from build123d import *

# Parameters (mm, degrees)
FLANGE_BASE1_DEPTH             = 3
CORTE_EXTRUS_O1_DEPTH          = 3
ARESTA_FLANGE4_STRIP_W         = 13.4732
ARESTA_FLANGE4_STRIP_H         = 3
ARESTA_FLANGE4_STRIP_CUT_DEPTH = 18.4
ARESTA_FLANGE4_DEPTH           = 18.4
ESBO_O47_W                     = 14.5
ESBO_O47_H                     = 15
RESSALTO_EXTRUS_O1_DEPTH       = 3
FILETE1_R                      = 5
ESBO_O48_W                     = 14.5
ESBO_O48_H                     = 15
RESSALTO_EXTRUS_O2_DEPTH       = 3
FILETE2_R                      = 5
FILETE3_R                      = 2
CORTE_EXTRUS_O5_DEPTH          = 42.850190918
CORTE_EXTRUS_O6_DEPTH          = 3


# Sheet-metal steps are written as plain solids
with BuildPart() as part:
    # Esboço1 → Flange-base1 (new body)
    with BuildSketch(Plane.XY):
        Polygon((-14.370772566, 2.693459119), (-4.370772566, 2.693459119), (-4.370772566, 5.943459119), (14.029227434, 5.943459119), (14.029227434, 2.693459119), (21.029227434, 2.693459119), (21.029227434, -4.306540881), (-14.370772566, -4.306540881), align=None)
    extrude(amount=-FLANGE_BASE1_DEPTH)

    # Esboço8 → Corte-extrusão1 (cut)
    with BuildSketch(Plane.XY):
        with BuildLine():
            Line((-10.260200759, 1.193459119), (-2.260200759, 1.193459119))
            ThreePointArc((-2.260200759, 1.193459119), (-0.260200759, -0.806540881), (-2.260200759, -2.806540881))
            Line((-2.260200759, -2.806540881), (-10.260200759, -2.806540881))
            ThreePointArc((-10.260200759, -2.806540881), (-12.260200759, -0.806540881), (-10.260200759, 1.193459119))
        make_face()
        with BuildLine():
            Line((8.88097681, 1.193459119), (17.620096532, 1.193459119))
            ThreePointArc((17.620096532, 1.193459119), (19.620096532, -0.806540881), (17.620096532, -2.806540881))
            Line((17.620096532, -2.806540881), (8.88097681, -2.806540881))
            ThreePointArc((8.88097681, -2.806540881), (6.88097681, -0.806540881), (8.88097681, 1.193459119))
        make_face()
    extrude(amount=-CORTE_EXTRUS_O1_DEPTH, mode=Mode.SUBTRACT)

    # Aresta-Flange4 strip (across the edge) → Aresta-Flange4 strip cut (cut)
    with BuildSketch(Plane(origin=(14.029227434, 5.943459119, 0), x_dir=(0, -1, 0), z_dir=(-1, 0, 0))):
        with Locations((-6, -1.5)):
            Rectangle(ARESTA_FLANGE4_STRIP_W, ARESTA_FLANGE4_STRIP_H)
    extrude(amount=ARESTA_FLANGE4_STRIP_CUT_DEPTH, mode=Mode.SUBTRACT)

    # Aresta-Flange4 section (across the edge) → Aresta-Flange4 (add)
    with BuildSketch(Plane(origin=(14.029227434, 5.943459119, 0), x_dir=(0, -1, 0), z_dir=(-1, 0, 0))):
        with BuildLine():
            Line((-3, 0.7366), (-3, 22.5))
            Line((-3, 22.5), (0, 22.5))
            Line((0, 22.5), (0, 0.7366))
            ThreePointArc((0, 0.7366), (0.215745145, 0.215745145), (0.7366, 0))
            Line((0.7366, 0), (0.7366, -3))
            ThreePointArc((0.7366, -3), (-1.905575199, -1.905575199), (-3, 0.7366))
        make_face()
    extrude(amount=ARESTA_FLANGE4_DEPTH)

    # Esboço47 → Ressalto-extrusão1 (add)
    with BuildSketch(Plane(origin=(14.029227434, 0, 0), x_dir=(0, 0, -1), z_dir=(1, 0, 0))):
        with Locations((-15.25, 13.443459119)):
            Rectangle(ESBO_O47_W, ESBO_O47_H)
    extrude(amount=-RESSALTO_EXTRUS_O1_DEPTH)

    # Filete1
    filete1_edges = [part.edges().sort_by_distance(p)[0] for p in [
        (12.529227434, 20.943459119, 22.5),
        (12.529227434, 8.943459119, 8),
        (12.529227434, 20.943459119, 8),
    ]]
    fillet(filete1_edges, radius=FILETE1_R)

    # Esboço48 → Ressalto-extrusão2 (add)
    with BuildSketch(Plane.ZY.offset(4.370772566)):
        with Locations((15.25, 13.443459119)):
            Rectangle(ESBO_O48_W, ESBO_O48_H)
    extrude(amount=-RESSALTO_EXTRUS_O2_DEPTH)

    # Filete2
    filete2_edges = [part.edges().sort_by_distance(p)[0] for p in [
        (-2.870772566, 20.943459119, 22.5),
        (-2.870772566, 8.943459119, 8),
        (-2.870772566, 20.943459119, 8),
    ]]
    fillet(filete2_edges, radius=FILETE2_R)

    # Filete3
    filete3_edges = [part.edges().sort_by_distance(p)[0] for p in [
        (21.029227434, -4.306540881, -1.5),
        (-14.370772566, -4.306540881, -1.5),
        (-14.370772566, 2.693459119, -1.5),
        (-4.370772566, 2.693459119, -1.5),
        (14.029227434, 2.693459119, -1.5),
        (21.029227434, 2.693459119, -1.5),
    ]]
    fillet(filete3_edges, radius=FILETE3_R)

    # Esboço49 → Corte-extrusão5 (cut, through all)
    with BuildSketch(Plane(origin=(14.029227434, 0, 0), x_dir=(0, 0, -1), z_dir=(1, 0, 0))):
        with BuildLine():
            Line((-18.2, 11.175198381), (-12.3, 11.175198381))
            ThreePointArc((-12.3, 11.175198381), (-10.885786438, 11.760984819), (-10.3, 13.175198381))
            Line((-10.3, 13.175198381), (-10.3, 17.289297618))
            ThreePointArc((-10.3, 17.289297618), (-10.885786438, 18.70351118), (-12.3, 19.289297618))
            Line((-12.3, 19.289297618), (-18.2, 19.289297618))
            ThreePointArc((-18.2, 19.289297618), (-19.614213562, 18.70351118), (-20.2, 17.289297618))
            Line((-20.2, 17.289297618), (-20.2, 13.175198381))
            ThreePointArc((-20.2, 13.175198381), (-19.614213562, 11.760984819), (-18.2, 11.175198381))
        make_face()
    extrude(amount=-CORTE_EXTRUS_O5_DEPTH, mode=Mode.SUBTRACT)

    # Esboço50 → Corte-extrusão6 (cut)
    with BuildSketch(Plane.XZ.offset(-5.943459119)):
        with BuildLine():
            Line((1.629227434, 19.2366), (8.029227434, 19.2366))
            ThreePointArc((8.029227434, 19.2366), (9.443440996, 18.650813562), (10.029227434, 17.2366))
            Line((10.029227434, 17.2366), (10.029227434, 5.2366))
            ThreePointArc((10.029227434, 5.2366), (9.443440996, 3.822386438), (8.029227434, 3.2366))
            Line((8.029227434, 3.2366), (1.629227434, 3.2366))
            ThreePointArc((1.629227434, 3.2366), (0.215013871, 3.822386438), (-0.370772566, 5.2366))
            Line((-0.370772566, 5.2366), (-0.370772566, 17.2366))
            ThreePointArc((-0.370772566, 17.2366), (0.215013871, 18.650813562), (1.629227434, 19.2366))
        make_face()
    extrude(amount=-CORTE_EXTRUS_O6_DEPTH, mode=Mode.SUBTRACT)


solid = part.part
Design review of the part built by this model. Coordinates are the model's own, in mm. A direction names the side the tool comes from. Coordinates: 2 decimals unless noted, no trailing zeros. Loops run counter-clockwise (first coordinate to the right, second up) from the corner with the lowest first, then second, coordinate; pieces in that order, holes last. Notation, with made-up numbers: M 50.5,20.25 L 91.5,20.25 A23 ccw 91.5,38.25 Z; hole C 64.5,42.25 d5. An arc over 180 degrees is marked long. Use one line per item in the form item = value.
(1) Consider section B-B (z = 15). Write out the cut boundary in (x, y).
Return value:
outline = M -4.37,5.94 L -0.37,5.94 L -0.37,8.94 L -1.37,8.94 L -1.37,11.18 L -4.37,11.18 Z; M -4.37,19.29 L -1.37,19.29 L -1.37,20.94 L -4.37,20.94 Z; M 10.03,5.94 L 14.03,5.94 L 14.03,11.18 L 11.03,11.18 L 11.03,8.94 L 10.03,8.94 Z; M 11.03,19.29 L 14.03,19.29 L 14.03,20.94 L 11.03,20.94 Z
(2) Consider section C-C (x = 4). Write out the cut boundary in (y, z).
Return value:
outline = M -4.31,-3 L 5.21,-3 A3.74 ccw 8.94,0.74 L 8.94,3.24 L 5.94,3.24 L 5.94,0.74 A0.74 cw 5.21,0 L -4.31,0 Z; M 5.94,19.24 L 8.94,19.24 L 8.94,22.5 L 5.94,22.5 Z
(3) Draft analysis for pull direction Z (two halves, no side actions). For faces 6 (the face through (21.029, -1, -1)), 7 (the face through (10.029, 7, 11)), 8 (the face through (12.508, 10.447, 6.574)), state which applies: pulls with the +Z half, pulls with the -Z half, needs draft (parallel to the pull), parting line crosses it, or undercut.
Return value:
face_6 = needs draft
face_7 = undercut
face_8 = pulls with the -Z half
(4) Clearance check with flat-ended pins moving along their axes: P1, Ø5, axis at y = 6.5, z = 2, coming from the +X side; P2, Ø10, axis at x = 8, z = 8.5, coming from the +Y side; P3, Ø10, axis at x = 11, z = 13.5, coming from the -Y side; P4, Ø14.5, axis at x = 3.5, z = 7, coming from the -Y side. State where each tip first meets the part, or that it passes through.
Return value:
P1 = 14.03
P2 = 20.92
P3 = 5.94
P4 = -4.31
(5) For faces 1 (the face through (-6, -2.807, -1)), 2 (the face through (11.029, 11, 15)), 3 (the face through (13, 15, 10.3)), 4 (the face through (9.46, 7.42, 3.84)), 5 (the face through (-9, 2.693, -1)), list the 3-axis set-ups (+Z, -Z, +X, -X, +Y, -Y) from which the entire face can be reached by the end or side of a thin tool; tool diameter is ignored.
Return value:
face_1 = +Z, -Z
face_2 = +Z, -Z, +Y
face_3 = +X, -X
face_4 = +Y, -Y
face_5 = +Z, -Z, -X, +Y
(6) Consider section A-A (x = 11.5). Write out the cut boundary in (y, z).
Return value:
outline = M -4.31,-3 L -2.81,-3 L -2.81,0 L -4.31,0 Z; M 1.19,-3 L 5.21,-3 A3.74 ccw 8.94,0.74 L 8.94,3 A5 cw 13.94,8 L 15.94,8 A5 ccw 20.94,13 L 20.94,17.5 A5 ccw 15.94,22.5 L 5.94,22.5 L 5.94,0.74 A0.74 cw 5.21,0 L 1.19,0 Z; hole M 11.18,12.3 A2 ccw 13.18,10.3 L 17.29,10.3 A2 ccw 19.29,12.3 L 19.29,18.2 A2 ccw 17.29,20.2 L 13.18,20.2 A2 ccw 11.18,18.2 Z
(7) Consider section D-D (y = 14.5). Write out the cut boundary in (x, z), and give its area (3 significant figures).
Return value:
outline = M -4.37,8 L -1.37,8 L -1.37,10.3 L -4.37,10.3 Z; M -4.37,20.2 L -1.37,20.2 L -1.37,22.5 L -4.37,22.5 Z; M 11.03,8 L 14.03,8 L 14.03,10.3 L 11.03,10.3 Z; M 11.03,20.2 L 14.03,20.2 L 14.03,22.5 L 11.03,22.5 Z
area = 27.6 mm2
(8) For line 1 along Z through (x, y) = (-2.5, 14.25); line 2 along Y through (x, z) = (-2, 17.5); line 3 along X through (y, z) = (8.5, 8.25), list the stretches that pass through material, from the lowest coordinate up. Write a range as from..to.
Return value:
line_1 = 8..10.3, 20.2..22.5
line_2 = 5.94..11.18, 19.29..20.94
line_3 = -4.37..-0.37, 10.03..14.03
